Source: CAD feature listing. Evaluate the final solid. Frame: model axes, mm. A direction names the side the tool comes from. Round coordinates to 2 decimals unless told otherwise and drop trailing zeros. Write each loop counter-clockwise with the first axis right and the second up, starting at its lowest first coordinate (ties: lowest second). Pieces come first, ordered by that corner, then holes. Notation, with made-up numbers: M 48.5,27.25 L 75.5,27.25 A25 cw 75.5,64.25 Z; hole C 20.25,63 d11. An arc over 180 degrees is marked long. Answer in a Markdown table with one row per item.
Autodesk Inventor part; units mm, degrees
ref_plane "YZ Plane" through (0, 0, 0) normal (1, 0, 0) x (0, 1, 0)
ref_plane "XZ Plane" through (0, 0, 0) normal (0, 1, 0) x (-1, 0, 0)
ref_plane "XY Plane" through (0, 0, 0) normal (0, 0, 1) x (1, 0, 0)
sketch "Sketch1" plane through (0, 0, 0) normal (0, 0, 1) x (1, 0, 0)
  line L0 (0, 0) -> (0, 30)
  line L1 (0, 30) -> (19, 30)
  line L2 (19, 30) -> (38, 5)
  line L3 (38, 5) -> (38, 0)
  line L4 (38, 0) -> (0, 0)
  dimension "C" = 76
  dimension "d1" = 30
  dimension "d2" = 5
  dimension "d3" = 38
revolve "Revolution1" add sketch "Sketch1" angle 360 about axis through (0, 0, 0) along (0, 1, 0)
shell "Shell1" thickness 5 removed faces 1 at (9.1519, 0, -15.3991)
sketch "Sketch2" plane through (0, 30, 0) normal (0, 1, 0) x (1, 0, 0)
  circle A0 centre (0, 0) radius 19
  circle A1 centre (0, 0) radius 6
  dimension "d6" = 12
extrude "Extrusion1" add sketch "Sketch2" along normal blind 50 contours A1
thread "Thread1"
equation "\"d3\" = 0.5 * C"
equation "\"d7\" = Dmax - d1"
equation "\"Dmin\" = 41"
equation "\"Dmax\" = 80"
properties part number "21-013"
Q1. Section C-C (y = 12). Return loops of the section in (x, z), and give its area (3 significant figures).
Solutions:
| item | result |
|---|---|
| outline | C 0,0 d65.36; hole C 0,0 d52.8 |
| area | 1,170 mm2 |
Q2. Contact query for flat-ended pins moving along their axis: pin 1 Ø1 at (x, y) = (18.5, 23) entering from +Z; pin 2 Ø5 at (x, z) = (-6, -30.5) entering from -Y; pin 3 Ø6 at (y, z) = (22, -21) entering from +X; pin 4 Ø6 at (x, z) = (-26.5, -19.5) entering from +Y. Output: stop coordinate, or through.
Solutions:
| item | result |
|---|---|
| pin 1 | stops at z = 16.59 |
| pin 2 | stops at y = 0 |
| pin 3 | stops at x = 18.87 |
| pin 4 | stops at y = 15.66 |
Q3. Section A-A (z = 0). Return loops of the section in (x, y).
Solutions:
| item | result |
|---|---|
| outline | M -38,0 L -33,0 L -33,3.32 L -16.52,25 L 16.52,25 L 33,3.32 L 33,0 L 38,0 L 38,5 L 19,30 L 6,30 L 6,80 L -6,80 L -6,30 L -19,30 L -38,5 Z |
Q4. Section D-D (y = 31.5). Return loops of the section in (x, z), and give its area (3 significant figures).
Solutions:
| item | result |
|---|---|
| outline | C 0,0 d12 |
| area | 113 mm2 |
Q5. Pull-direction query (X, two-part tool) for faces 1 (the cylindrical face through (-6, 55, 0)), 2 (the flat face through (0, 80, 0)), 3 (the flat face through (0, 25, 0)); classes: pulls with the +X half, pulls with the -X half, needs draft (parallel to the pull), parting line crosses it, or undercut.
Solutions:
| item | result |
|---|---|
| face 1 | parting line crosses it |
| face 2 | needs draft |
| face 3 | undercut |
Q6. Material intervals for probe 1 along Z at (x, y) = (0, 1); probe 2 along Z at (x, y) = (2.5, 6.5); probe 3 along Y at (x, z) = (-1, -13), sorted ascending.
Solutions:
| item | result |
|---|---|
| probe 1 | z = -38 to -33, 33 to 38 |
| probe 2 | z = -36.78 to -30.48, 30.48 to 36.78 |
| probe 3 | y = 25 to 30 |
Q7. Access query for faces 4 (the cylindrical face through (17.535, 2.465, -33.713)), 5 (the cylindrical face through (30.5, 1.6, -12.6)), 6 (the flat face through (-4.5, 30, -4.5)). Directions: +Z, -Z, +X, -X, +Y, -Y. A direction counts if a zero-diameter tool reaches every point of the face in a straight line with its end or side. Return the directions, or none.
Solutions:
| item | result |
|---|---|
| face 4 | +Y, -Y |
| face 5 | -Y |
| face 6 | +Y |
Q8. Section B-B (x = 0). Return loops of the section in (y, z), and give its area (3 significant figures).
Solutions:
| item | result |
|---|---|
| outline | M 0,-38 L 5,-38 L 30,-19 L 30,-6 L 80,-6 L 80,6 L 30,6 L 30,19 L 5,38 L 0,38 L 0,33 L 3.32,33 L 25,16.52 L 25,-16.52 L 3.32,-33 L 0,-33 Z |
| area | 1,110 mm2 |
